```python
from build123d import *

# Parameters (mm, degrees)
F0_R      = 6.35
F1_DEPTH  = 25.4
F2_R      = 9.525
F3_DEPTH  = 25.4
F4_R      = 12.7
F5_DEPTH  = 25.4
F6_R      = 15.875
F7_DEPTH  = 25.4
F8_R      = 19.05
F9_DEPTH  = 25.4
F10_R     = 22.225
F11_DEPTH = 25.4
F12_R     = 25.4
F13_DEPTH = 25.4


with BuildPart() as f1:
    # F0 (on Front) → F1 (new body)
    with BuildSketch(Plane.XZ):
        Circle(F0_R)
    extrude(amount=F1_DEPTH)

    # F2 (on face) → F3 (join)
    with BuildSketch(Plane.XZ.offset(25.4)):
        Circle(F2_R)
    extrude(amount=F3_DEPTH)

    # F4 (on face) → F5 (join)
    with BuildSketch(Plane.XZ.offset(50.8)):
        Circle(F4_R)
    extrude(amount=F5_DEPTH)

    # F6 (on face) → F7 (join)
    with BuildSketch(Plane.XZ.offset(76.2)):
        Circle(F6_R)
    extrude(amount=F7_DEPTH)

    # F8 (on face) → F9 (join)
    with BuildSketch(Plane.XZ.offset(101.6)):
        Circle(F8_R)
    extrude(amount=F9_DEPTH)

    # F10 (on face) → F11 (join)
    with BuildSketch(Plane.XZ.offset(127)):
        Circle(F10_R)
    extrude(amount=F11_DEPTH)

    # F12 (on face) → F13 (join)
    with BuildSketch(Plane.XZ.offset(152.4)):
        Circle(F12_R)
    extrude(amount=F13_DEPTH)


solid = f1.part
```
Can you work these out from the model? Positions are in its coordinate system, mm. A direction names the side the tool comes from. Give positions to 0.01 mm unless a question says otherwise; leave off trailing zeros. Order: outer loops, then holes, each group sorted by start corner. A loop starts at its lowest first (then second) coordinate and runs counter-clockwise, first axis right, second up. Notation, with made-up numbers: M 8,-37.75 L 32,-37.75 A22 ccw 32,-25.75 Z; hole C -31.5,-6.5 d2. An arc over 180 degrees is marked long. Write item = value, one per line. Start each with the question number.
Q1. For faces 1 (the flat face through (-0.1, -152.4, -22.5)), 2 (the flat face through (0, -177.8, 0)), which set-ups out of +Z, -Z, +X, -X, +Y, -Y let a thin tool reach every point of the face, with its end or its side?
Q2. Suppose I cut it at D-D (y = -29.5). Write out the boundary of the cut face in (x, z) (3 decimals), plus the area to 3 significant figures.
Q3. Suppose I cut it at A-A (x = 0). Write out the boundary of the cut face in (y, z) (3 decimals).
Q4. Will these pins go through, and if not, where does the flat tip stop? pin 1 Ø2 at (x, y) = (0.5, -45) entering from -Z (3 decimals); pin 2 Ø3 at (x, y) = (-13.5, -85.5) entering from -Z; pin 3 Ø6 at (x, y) = (-8, -55.5) entering from +Z.
Q5. Suppose I cut it at B-B (z = 0). Write out the boundary of the cut face in (x, y) (3 decimals).
Q6. I need wall thicknesses on probe 1 along Y at (x, z) = (14, -7); probe 2 along Y at (x, z) = (-14, -21); probe 3 along Z at (x, y) = (11, -56). Which ranges of each line are inside material? Lowest first, please. Write a range as [from, to].
Q7. Suppose I cut it at C-C (y = -94). Write out the boundary of the cut face in (x, z) (3 decimals).
Check result:
q1.face_1 = +Y
q1.face_2 = +Z, -Z, +X, -X, -Y
q2.outline = C 0,0 d19.05
q2.area = 285 mm2
q3.outline = M -177.8,-25.4 L -152.4,-25.4 L -152.4,-22.225 L -127,-22.225 L -127,-19.05 L -101.6,-19.05 L -101.6,-15.875 L -76.2,-15.875 L -76.2,-12.7 L -50.8,-12.7 L -50.8,-9.525 L -25.4,-9.525 L -25.4,-6.35 L 0,-6.35 L 0,6.35 L -25.4,6.35 L -25.4,9.525 L -50.8,9.525 L -50.8,12.7 L -76.2,12.7 L -76.2,15.875 L -101.6,15.875 L -101.6,19.05 L -127,19.05 L -127,22.225 L -152.4,22.225 L -152.4,25.4 L -177.8,25.4 Z
q4.pin_1 = -9.525
q4.pin_2 = -10.39
q4.pin_3 = 11.67
q5.outline = M -25.4,-177.8 L 25.4,-177.8 L 25.4,-152.4 L 22.225,-152.4 L 22.225,-127 L 19.05,-127 L 19.05,-101.6 L 15.875,-101.6 L 15.875,-76.2 L 12.7,-76.2 L 12.7,-50.8 L 9.525,-50.8 L 9.525,-25.4 L 6.35,-25.4 L 6.35,0 L -6.35,0 L -6.35,-25.4 L -9.525,-25.4 L -9.525,-50.8 L -12.7,-50.8 L -12.7,-76.2 L -15.875,-76.2 L -15.875,-101.6 L -19.05,-101.6 L -19.05,-127 L -22.225,-127 L -22.225,-152.4 L -25.4,-152.4 Z
q6.probe_1 = [-177.8, -76.2]
q6.probe_2 = [-177.8, -152.4]
q6.probe_3 = [-6.35, 6.35]
q7.outline = C 0,0 d31.75
